```python
from build123d import *

# Parameters (mm, degrees)
SKETCH1_W                       = 62.15
SKETCH1_H                       = 78
BOSS_EXTRUDE1_DEPTH             = 9
SPRING_PULLEY_CUTOUT_DEPTH      = 10
SPRING_PULLEY_CUTOUT_DEPTH_BACK = 11.2
SKETCH2_R                       = 25
SKETCH3_R                       = 1.225
CUT_EXTRUDE2_DEPTH              = 7.5
SKETCH4_R                       = 0.75
CUT_EXTRUDE3_DEPTH              = 101.014361469
CHAMFER1_SIZE                   = 0.4
CHAMFER1_SIZE2                  = 0.692820323
MOTOR_HOLDER_DEPTH              = 32.95
MOVE_FACE7_BY                   = 0.4
SKETCH20_R                      = 2.55
CUT_EXTRUDE8_DEPTH              = 7
BOSS_EXTRUDE5_DEPTH             = 32.55
MOVE_FACE3_BY                   = 1
CUT_EXTRUDE12_DEPTH             = 108.086985671
FILLET12_R                      = 1.8
SKETCH24_R                      = 1.6
MOTOR_CLIP_HOLES_DEPTH          = 3
SKETCH26_W                      = 5.75
SKETCH26_H                      = 12.7
CUT_EXTRUDE13_DEPTH             = 110.829970864
SKETCH27_R                      = 2
CUT_EXTRUDE14_DEPTH             = 7.25
SKETCH29_R                      = 0.8
CUT_EXTRUDE16_DEPTH             = 5
SKETCH52_W                      = 78
SKETCH52_H                      = 9
CUT_EXTRUDE31_DEPTH             = 7.25
MOVE_START                      = -54.4
MOVE_FACE6_OUTLINE_W            = 5.75
MOVE_FACE6_OUTLINE_H            = 9
MOVE_FACE6_DEPTH                = 13.1
SKETCH31_W                      = 2
SKETCH31_H                      = 4
SKETCH32_R                      = 3
CUT_EXTRUDE17_DEPTH             = 105.439563953
MOTOR_CLIP_WIRE_FILLET_R        = 2
BOSS_EXTRUDE8_DEPTH             = 9
FILLET13_R                      = 1.5
M5_CLEARANCE_HOLE1_D            = 5.5


# Read off the part's stored shape, not the designer's step: Move Face6
with BuildPart() as part:
    # Sketch1 → Boss-Extrude1 (new body)
    with BuildSketch(Plane(origin=(0, 0, 0), x_dir=(1, 0, 0), z_dir=(0, 1, 0))):
        with Locations((31.075, 39)):
            Rectangle(SKETCH1_W, SKETCH1_H)
    extrude(amount=BOSS_EXTRUDE1_DEPTH)

    # Sketch2 → spring_pulley_cutout (cut, two sides: drawn at the far end of the back side and taken through both)
    with BuildSketch(Plane.ZY.offset(-18).offset(-SPRING_PULLEY_CUTOUT_DEPTH_BACK)):
        with Locations((-24, -18)):
            Circle(SKETCH2_R)
    extrude(amount=SPRING_PULLEY_CUTOUT_DEPTH + SPRING_PULLEY_CUTOUT_DEPTH_BACK, mode=Mode.SUBTRACT)

    # Sketch3 → Cut-Extrude2 (cut)
    with BuildSketch(Plane(origin=(0, 9, 0), x_dir=(1, 0, 0), z_dir=(0, 1, 0))):
        with Locations(Location((12.85, 4, 0), (0, 0, 270))):
            Circle(SKETCH3_R)
        with Locations(Location((23.15, 44, 0), (0, 0, 270))):
            Circle(SKETCH3_R)
    extrude(amount=-CUT_EXTRUDE2_DEPTH, mode=Mode.SUBTRACT)

    # Sketch4 → Cut-Extrude3 (cut, through all)
    with BuildSketch(Plane(origin=(0, 1.5, 0), x_dir=(1, 0, 0), z_dir=(0, 1, 0))):
        with Locations(Location((12.85, 4, 0), (0, 0, 270))):
            Circle(SKETCH4_R)
        with Locations(Location((23.15, 44, 0), (0, 0, 270))):
            Circle(SKETCH4_R)
    extrude(amount=-CUT_EXTRUDE3_DEPTH, mode=Mode.SUBTRACT)

    # Chamfer1
    chamfer1_edges = [part.edges().sort_by_distance(p)[0] for p in [
        (12.85, 9, -5.225),
        (23.15, 9, -45.225),
    ]]
    chamfer1_side = [part.faces().sort_by_distance(p)[0] for p in [
        (31.100480241, 9, -39.029231634),
    ]]
    chamfer(chamfer1_edges, length=CHAMFER1_SIZE, length2=CHAMFER1_SIZE2, reference=chamfer1_side[0])

    # Sketch19 → Motor Holder (add)
    with BuildSketch(Plane.ZY.offset(-29.2)):
        with BuildLine():
            Line((-54.8, -18), (-38, -18))
            ThreePointArc((-38, -18), (-24, -4), (-10, -18))
            Line((-10, -18), (0, -18))
            Line((0, -18), (0, 0))
            Line((0, 0), (-54.8, 0))
            Line((-54.8, 0), (-54.8, -18))
        make_face()
    extrude(amount=-MOTOR_HOLDER_DEPTH)

    # Move Face7: a face moved inward by 0.4
    extrude(part.faces().sort_by_distance((29.2, 0.75, -27.4))[0], amount=MOVE_FACE7_BY, dir=(1, 0, 0), mode=Mode.SUBTRACT)

    # Sketch20 → Cut-Extrude8 (cut)
    with BuildSketch(Plane(origin=(0, -18, 0), x_dir=(-1, 0, 0), z_dir=(0, -1, 0))):
        with Locations(Location((-57.15, 5, 0), (0, 0, 90))):
            Circle(SKETCH20_R)
        with Locations(Location((-34.6, 5, 0), (0, 0, 90))):
            Circle(SKETCH20_R)
        with Locations(Location((-57.15, 46.4, 0), (0, 0, 90))):
            Circle(SKETCH20_R)
        with Locations(Location((-34.6, 46.4, 0), (0, 0, 90))):
            Circle(SKETCH20_R)
    extrude(amount=-CUT_EXTRUDE8_DEPTH, mode=Mode.SUBTRACT)

    # Move Face3: a face moved inward by 1.0
    extrude(part.faces().sort_by_distance((8, 2.836578696, -24))[0], amount=MOVE_FACE3_BY, dir=(-1, 0, 0), mode=Mode.SUBTRACT)

    # Sketch26 → Cut-Extrude13 (cut, through all)
    with BuildSketch(Plane(origin=(0, 9, 0), x_dir=(1, 0, 0), z_dir=(0, 1, 0))):
        with Locations((10.125, 47.85)):
            Rectangle(SKETCH26_W, SKETCH26_H)
    extrude(amount=-CUT_EXTRUDE13_DEPTH, mode=Mode.SUBTRACT)

    # Sketch27 → Cut-Extrude14 (cut)
    with BuildSketch(Plane.ZY):
        with Locations((-44.6, 5)):
            Circle(SKETCH27_R)
        with Locations((-51.1, 5)):
            Circle(SKETCH27_R)
    extrude(amount=-CUT_EXTRUDE14_DEPTH, mode=Mode.SUBTRACT)

    # Sketch29 → Cut-Extrude16 (cut)
    with BuildSketch(Plane.ZY.offset(-13)):
        with Locations((-51.1, 5)):
            Circle(SKETCH29_R)
        with Locations((-44.6, 5)):
            Circle(SKETCH29_R)
    extrude(amount=-CUT_EXTRUDE16_DEPTH, mode=Mode.SUBTRACT)

    # Sketch52 → Cut-Extrude31 (cut)
    with BuildSketch(Plane.ZY):
        with Locations((-39, 4.5)):
            Rectangle(SKETCH52_W, SKETCH52_H)
    extrude(amount=-CUT_EXTRUDE31_DEPTH, mode=Mode.SUBTRACT)

    # Move Face6 outline → Move Face6 (cut)
    with BuildSketch(Plane.XY.offset(MOVE_START)):
        with Locations((10.125, 4.5)):
            Rectangle(MOVE_FACE6_OUTLINE_W, MOVE_FACE6_OUTLINE_H)
    extrude(amount=MOVE_FACE6_DEPTH, mode=Mode.SUBTRACT)

    # Cut-Sweep1: sweep along a path in Sketch30
    with BuildLine(Plane(origin=(0, -12, 0), x_dir=(-1, 0, 0), z_dir=(0, -1, 0))) as cut_sweep1_path:
        CenterArc((-45.875, 0), 5, 0, 360)
    # Sketch31 → Cut-Sweep1 (sweep, cut)
    with BuildSketch(Plane(origin=(0, 0, 0), x_dir=(-1, 0, 0), z_dir=(0, 0, -1))):
        with Locations((-42.875, -12)):
            Rectangle(SKETCH31_W, SKETCH31_H)
    sweep(path=cut_sweep1_path.line, mode=Mode.SUBTRACT)


with BuildPart() as body_2:
    # Sketch22 → Boss-Extrude5 (new body)
    with BuildSketch(Plane.ZY.offset(-29.6)):
        with BuildLine():
            Line((0, -19), (-10.035759956, -19))
            ThreePointArc((-10.035759956, -19), (-24, -32), (-37.964240044, -19))
            Line((-37.964240044, -19), (-54.8, -19))
            Line((-54.8, -19), (-54.8, -39))
            Line((-54.8, -39), (0, -39))
            Line((0, -39), (0, -19))
        make_face()
    extrude(amount=-BOSS_EXTRUDE5_DEPTH)

    # Sketch25 → Cut-Extrude12 (cut, through all)
    with BuildSketch(Plane(origin=(62.15, 0, 0), x_dir=(0, 0, -1), z_dir=(1, 0, 0))):
        with BuildLine():
            Line((54.8, -22), (42.574175621, -22))
            ThreePointArc((42.574175621, -22), (24, -37), (5.425824379, -22))
            Line((5.425824379, -22), (0, -22))
            Line((0, -22), (0, -42))
            Line((0, -42), (54.8, -42))
            Line((54.8, -42), (54.8, -22))
        make_face()
    extrude(amount=-CUT_EXTRUDE12_DEPTH, mode=Mode.SUBTRACT)

    # Fillet12
    fillet12_edges = [body_2.edges().sort_by_distance(p)[0] for p in [
        (62.15, -20.5, 0),
        (62.15, -20.5, -54.8),
        (29.6, -20.5, 0),
        (45.875, -22, -5.425824379),
        (45.875, -22, -42.574175621),
        (29.6, -20.5, -54.8),
    ]]
    fillet(fillet12_edges, radius=FILLET12_R)

    # Sketch24 → Motor Clip Holes (cut)
    with BuildSketch(Plane.XZ.offset(22)):
        with Locations(Location((34.6, -5, 0), (0, 0, 37.543618534))):
            Circle(SKETCH24_R)
        with Locations(Location((57.15, -5, 0), (0, 0, 37.543618534))):
            Circle(SKETCH24_R)
        with Locations(Location((34.6, -46.4, 0), (0, 0, 270))):
            Circle(SKETCH24_R)
        with Locations(Location((57.15, -46.4, 0), (0, 0, 270))):
            Circle(SKETCH24_R)
    extrude(amount=-MOTOR_CLIP_HOLES_DEPTH, mode=Mode.SUBTRACT)

    # Sketch32 → Cut-Extrude17 (cut, through all)
    with BuildSketch(Plane.XZ.offset(22)):
        with Locations((57.15, -5)):
            Circle(SKETCH32_R)
        with Locations((57.15, -46.4)):
            Circle(SKETCH32_R)
        with Locations((34.6, -46.4)):
            Circle(SKETCH32_R)
        with Locations((34.6, -5)):
            Circle(SKETCH32_R)
    extrude(amount=CUT_EXTRUDE17_DEPTH, mode=Mode.SUBTRACT)

    # Motor Clip Wire Fillet
    # the kernel refuses this fillet: 2 mm, written as the material it takes off along each edge
    with BuildSketch(Plane(origin=(29.6, -18, -24), x_dir=(0, -0.27884615384615374, 0.9603357863191433), z_dir=(0, 0.9603357863191433, 0.27884615384615374))) as motor_clip_wire_fillet_piece_1:
        with BuildLine():
            CenterArc((19 - MOTOR_CLIP_WIRE_FILLET_R, MOTOR_CLIP_WIRE_FILLET_R), MOTOR_CLIP_WIRE_FILLET_R, 270, 90)
            Line((19 - MOTOR_CLIP_WIRE_FILLET_R, 0), (19, 0))
            Line((19, 0), (19, MOTOR_CLIP_WIRE_FILLET_R))
        make_face()
    revolve(axis=Axis((29.6, -18, -24), (1, 0, 0)), revolution_arc=147.617296723, mode=Mode.SUBTRACT)
    with BuildSketch(Plane(origin=(29.6, -23.8, -43.974984355), x_dir=(0, 0.2788461538461544, 0.960335786319143), z_dir=(0, -0.960335786319143, 0.2788461538461544))) as motor_clip_wire_fillet_piece_2:
        with BuildLine():
            CenterArc((1.8 + MOTOR_CLIP_WIRE_FILLET_R, -MOTOR_CLIP_WIRE_FILLET_R), MOTOR_CLIP_WIRE_FILLET_R, 90, 90)
            Line((1.8 + MOTOR_CLIP_WIRE_FILLET_R, 0), (1.8, 0))
            Line((1.8, 0), (1.8, -MOTOR_CLIP_WIRE_FILLET_R))
        make_face()
    revolve(axis=Axis((29.6, -23.8, -43.974984355), (-1, 0, 0)), revolution_arc=233.006586684, mode=Mode.SUBTRACT)
    with BuildSketch(Plane(origin=(29.6, -23.8, -4.025015645), x_dir=(0, -0.9348128979547861, 0.3551406000690075), z_dir=(0, -0.3551406000690075, -0.9348128979547861))) as motor_clip_wire_fillet_piece_3:
        with BuildLine():
            CenterArc((1.8 + MOTOR_CLIP_WIRE_FILLET_R, -MOTOR_CLIP_WIRE_FILLET_R), MOTOR_CLIP_WIRE_FILLET_R, 90, 90)
            Line((1.8 + MOTOR_CLIP_WIRE_FILLET_R, 0), (1.8, 0))
            Line((1.8, 0), (1.8, -MOTOR_CLIP_WIRE_FILLET_R))
        make_face()
    revolve(axis=Axis((29.6, -23.8, -4.025015645), (-1, 0, 0)), revolution_arc=233.006586684, mode=Mode.SUBTRACT)

    # Sketch64 → Boss-Extrude8 (add)
    with BuildSketch(Plane(origin=(62.15, 0, 0), x_dir=(0, 0, -1), z_dir=(1, 0, 0))):
        with BuildLine():
            Line((8, -28.246950766), (8, -60.2))
            Line((8, -60.2), (42.24637994, -60.2))
            Line((42.24637994, -60.2), (42.24637994, -23.298076923))
            ThreePointArc((42.24637994, -23.298076923), (26.717424109, -36.804669798), (8, -28.246950766))
        make_face()
    extrude(amount=-BOSS_EXTRUDE8_DEPTH)

    # Fillet13
    fillet13_edges = [body_2.edges().sort_by_distance(p)[0] for p in [
        (57.65, -60.2, -42.24637994),
        (57.65, -60.2, -8),
    ]]
    fillet(fillet13_edges, radius=FILLET13_R)

    # M5 Clearance Hole1 (through all)
    with Locations(Plane(origin=(62.15, 0, 0), x_dir=(0, 0, -1), z_dir=(1, 0, 0))):
        with Locations((16, -50.2), (34.24637994, -50.2)):
            Hole(M5_CLEARANCE_HOLE1_D / 2)


solid = body_2.part
```
For this review, take the finished solid that the model builds, in its own axes (mm). A direction names the side the tool comes from. Coordinates: 2 decimals unless noted, no trailing zeros. Write each loop counter-clockwise with the first axis right and the second up, starting at its lowest first coordinate (ties: lowest second). Pieces come first, ordered by that corner, then holes.
(1) The part is to be moulded in two halves that separate along X. For faces 3 (the face through (62.15, -39, -27)), 4 (the face through (57.1, -24.4, -8)), 5 (the face through (53.15, -46, -25)), 6 (the face through (58, -43, -8)), say which applies: +X half, -X half, draft (parallel to the pull), parting line (faces both ways), or undercut.
(2) Tool access review of faces 1 (the face through (58, -41, -42.246)), 2 (the face through (46, -32, -24)): name each direction out of +Z, -Z, +X, -X, +Y, -Y from which nothing blocks a thin tool from reaching the whole face with its end or side.
(3) Wall thickness on probe 1 along X at (y, z) = (-19.7, -5); probe 2 along Z at (x, y) = (56, -50); probe 3 along Z at (x, y) = (40.5, -21): over which ranges is each line inside the solid? List them lowest first.
(4) Add section D-D on y = -43. Give the boundary of the cut face in (x, z).
(5) Add section C-C on z = -46.4. Count the separate pieces of the cut face and the enclosed holes in it, then the cut area to 3 significant figures.
(6) For pin 1 Ø8 at (x, y) = (55.5, -35) entering from +Z; pin 2 Ø5 at (x, y) = (48.5, -28.5) entering from +Z; pin 3 Ø7 at (y, z) = (-50.2, -34.25) entering from +X; pin 4 Ø1.5 at (x, z) = (57.5, -14.5) entering from +Y, all flat-tipped, find the tip position at first contact; note any pin that passes through.
(7) Add section B-B on x = 34.6. Give the boundary of the cut face in (y, z), then the cut area to 3 significant figures.
(8) Add section A-A on y = -50.2. Give the boundary of the cut face in (x, z), then the cut area to 3 significant figures.
Answer sheet:
1. face 3: +X half
1. face 4: undercut
1. face 5: -X half
1. face 6: draft
2. face 1: -Z, +X, -X, -Y
2. face 2: +X, -X, +Y
3. probe 1: x = 29.6 to 33, 36.2 to 55.55, 58.75 to 62.15
3. probe 2: z = -42.25 to -36.99, -31.5 to -18.74, -13.26 to -8
3. probe 3: z = -54.8 to -37.67, -10.33 to 0
4. outline: (53.15, -42.25) - (62.15, -42.25) - (62.15, -8) - (53.15, -8) - close
5. separate pieces: 3
5. enclosed holes: 0
5. area: 78.4 mm2
6. pin 1: stops at z = -8
6. pin 2: stops at z = -6.77
6. pin 3: stops at x = 62.15
6. pin 4: stops at y = -27.54
7. outline: (-28.25, -8) arc R19 ccw to (-23.3, -42.25) arc R1.8 cw to (-22.09, -43.4) - (-22, -43.4) - (-22, -44.8) - (-19, -44.8) - (-19, -37.96) arc R14 cw to (-19, -10.04) - (-19, -6.6) - (-22, -6.6) - (-22, -8) - close; (-22, -54.8) - (-19, -54.8) - (-19, -48) - (-22, -48) - close; (-22, -3.4) - (-19, -3.4) - (-19, 0) - (-22, 0) - close
7. area: 272 mm2
8. outline: (53.15, -42.25) - (62.15, -42.25) - (62.15, -37) - (53.15, -37) - close; (53.15, -31.5) - (62.15, -31.5) - (62.15, -18.75) - (53.15, -18.75) - close; (53.15, -13.25) - (62.15, -13.25) - (62.15, -8) - (53.15, -8) - close
8. area: 209 mm2
